CAD build for the part. Positions are in the model's coordinates, mm. A direction names the side the tool comes from. Coordinates: 2 decimals unless noted, no trailing zeros. Loops run counter-clockwise (first coordinate to the right, second up) from the corner with the lowest first, then second, coordinate; pieces in that order, holes last. Notation, with made-up numbers: (-28, 69) - (28, 69) arc R20 ccw to (28, 89) - close; hole circle Ø3 at (-19, 15.5). An arc over 180 degrees is marked (long way). Put each result on its own line as item: value.
```python
from build123d import *

# Parameters (mm, degrees)
SKETCH_1_R               = 47.5
EXTRUDE_1_DEPTH          = 80
CUT_EXTRUDE_START        = -40
CUT_EXTRUDE_1_DEPTH      = 40
FILLET_1_R               = 5
SKETCH_3_R               = 12.5
CUT_EXTRUDE_2_DEPTH      = 115.945639495
CHAMFER_1_SIZE           = 1
CUT_EXTRUDE_3_DEPTH      = 105.462912246
CUT_EXTRUDE_3_DEPTH_BACK = 105.462912246
SKETCH_4_R               = 10


with BuildPart() as part:
    # Эскиз1 → Бобышка-Вытянуть1 (new body)
    with BuildSketch(Plane.XY):
        Circle(SKETCH_1_R)
    extrude(amount=EXTRUDE_1_DEPTH)

    # Эскиз2 → Вырез-Вытянуть1 (cut)
    with BuildSketch(Plane.XY.offset(80).offset(CUT_EXTRUDE_START)):
        with BuildLine():
            Line((20, -43.084219849), (20, 43.084219849))
            ThreePointArc((20, 43.084219849), (47.5, 0), (20, -43.084219849))
        make_face()
        with BuildLine():
            Line((-20, -43.084219849), (-20, 43.084219849))
            ThreePointArc((-20, 43.084219849), (-47.5, 0), (-20, -43.084219849))
        make_face()
    extrude(amount=CUT_EXTRUDE_1_DEPTH, mode=Mode.SUBTRACT)

    # Скругление1
    fillet_1_edges = [part.edges().sort_by_distance(p)[0] for p in [
        (-20, 0, 40),
        (20, 0, 40),
    ]]
    fillet(fillet_1_edges, radius=FILLET_1_R)

    # Эскиз3 → Вырез-Вытянуть2 (cut, through all)
    with BuildSketch(Plane.ZY.offset(20)):
        with Locations(Location((55, 0, 0), (0, 0, 216.869897646))):
            Circle(SKETCH_3_R)
    extrude(amount=-CUT_EXTRUDE_2_DEPTH, mode=Mode.SUBTRACT)

    # Фаска1
    chamfer_1_edges = [part.edges().sort_by_distance(p)[0] for p in [
        (-20, 0, 80),
        (20, 0, 80),
    ]]
    chamfer(chamfer_1_edges, length=CHAMFER_1_SIZE)

    # Эскиз4 → Вырез-Вытянуть3 (cut, two sides: drawn at the far end of the back side and taken through both)
    with BuildSketch(Plane(origin=(0, 0, 0), x_dir=(0, 0, -1), z_dir=(1, 0, 0)).offset(-CUT_EXTRUDE_3_DEPTH_BACK)):
        with Locations((-15, 0)):
            Circle(SKETCH_4_R)
    extrude(amount=CUT_EXTRUDE_3_DEPTH + CUT_EXTRUDE_3_DEPTH_BACK, mode=Mode.SUBTRACT)


solid = part.part
```
Q1. Wall check: L1, parallel to Z at x = -0.5, y = 0; L2, parallel to Z at x = -39, y = 16.5; L3, parallel to X at y = -33, z = 74. Give the ranges that are in metal, low to high. Write a range as from..to.
Determined:
L1: 0..5, 25..42.5, 67.5..80
L2: 0..40
L3: -20..20
Q2. Slice it at C-C, the plane x = 0. Give the cut face in (y, z), then the cut area to 3 significant figures.
Determined:
outline: (-47.5, 0) - (47.5, 0) - (47.5, 80) - (-47.5, 80) - close; hole circle Ø25 at (0, 55); hole circle Ø20 at (0, 15)
area: 6,790 mm2
Q3. Slice it at B-B, the plane y = 0. Give the cut face in (x, z).
Determined:
outline: (-47.5, 0) - (47.5, 0) - (47.5, 5) - (-47.5, 5) - close; (-47.5, 25) - (47.5, 25) - (47.5, 40) - (25, 40) arc R5 cw to (20.67, 42.5) - (-20, 42.5) - (-20, 45) arc R5 cw to (-25, 40) - (-47.5, 40) - close; (-20, 67.5) - (20, 67.5) - (20, 79) - (19, 80) - (-19, 80) - (-20, 79) - close
Q4. Slice it at A-A, the plane z = 47.5. Give the cut face in (x, y), then the cut area to 3 significant figures.
Determined:
outline: (-20, -43.08) arc R47.5 ccw to (20, -43.08) - (20, -10) - (-20, -10) - close; (-20, 10) - (20, 10) - (20, 43.08) arc R47.5 ccw to (-20, 43.08) - close
area: 2,880 mm2
Q5. Tool access for faces 1 (the flat face through (0, 1, 80)), 2 (the flat face through (-20, 0, 43)), 3 (the flat face through (20, -1, 69)), 4 (the flat face through (-1, 1, 0)), 5 (the flat face through (-34, 1, 40)): list every direction of +Z, -Z, +X, -X, +Y, -Y with a clear straight run to the whole face (end or side of a thin tool).
Determined:
face 1: +Z, +X, -X, +Y, -Y
face 2: +X
face 3: +Z, +X, +Y, -Y
face 4: -Z, +X, -X, +Y, -Y
face 5: +Z, -X, +Y, -Y
Q6. Slice it at D-D, the plane x = 34. Give the cut face in (y, z), then the cut area to 3 significant figures.
Determined:
outline: (-33.17, 0) - (33.17, 0) - (33.17, 40) - (-33.17, 40) - close; hole circle Ø20 at (0, 15)
area: 2,340 mm2
Q7. Pin check, flat tips, straight feed: pin 1 Ø10 at (y, z) = (9, 67.5) entering from -X; pin 2 Ø12 at (y, z) = (4.5, 11.5) entering from +X; pin 3 Ø6 at (x, y) = (-25, -27) entering from +Z. Stop position of each tip, or through.
Determined:
pin 1: x = -20
pin 2: x = 47.38
pin 3: z = 41
Q8. Mould opens along Y. For faces 6 (the cylindrical face through (22, 1, 41)), 7 (the cylindrical face through (0.05, 7.05, 65.32)), 8 (the cylindrical face through (45.307, 14.268, 30.551)) say: +Y half, -Y half, draft (parallel to the pull), parting line (faces both ways), or undercut.
Determined:
face 6: draft
face 7: undercut
face 8: parting line
